Job drawing, mm, ordinate dimensions from the low corner. One solid piece. Coordinates: 2 decimals unless noted, no trailing zeros. Order: outer loops, then holes, each group sorted by start corner. A loop starts at its lowest first (then second) coordinate and runs counter-clockwise, first axis right, second up. Notation, with made-up numbers: (87.5, 36.5) - (93.5, 36.5) arc R23 ccw to (93.5, 69.5) - close; hole circle Ø7 at (-37.5, 64.5). An arc over 180 degrees is marked (long way). Write each question's results on one line, items separated by ' | '. Start each with the question number.
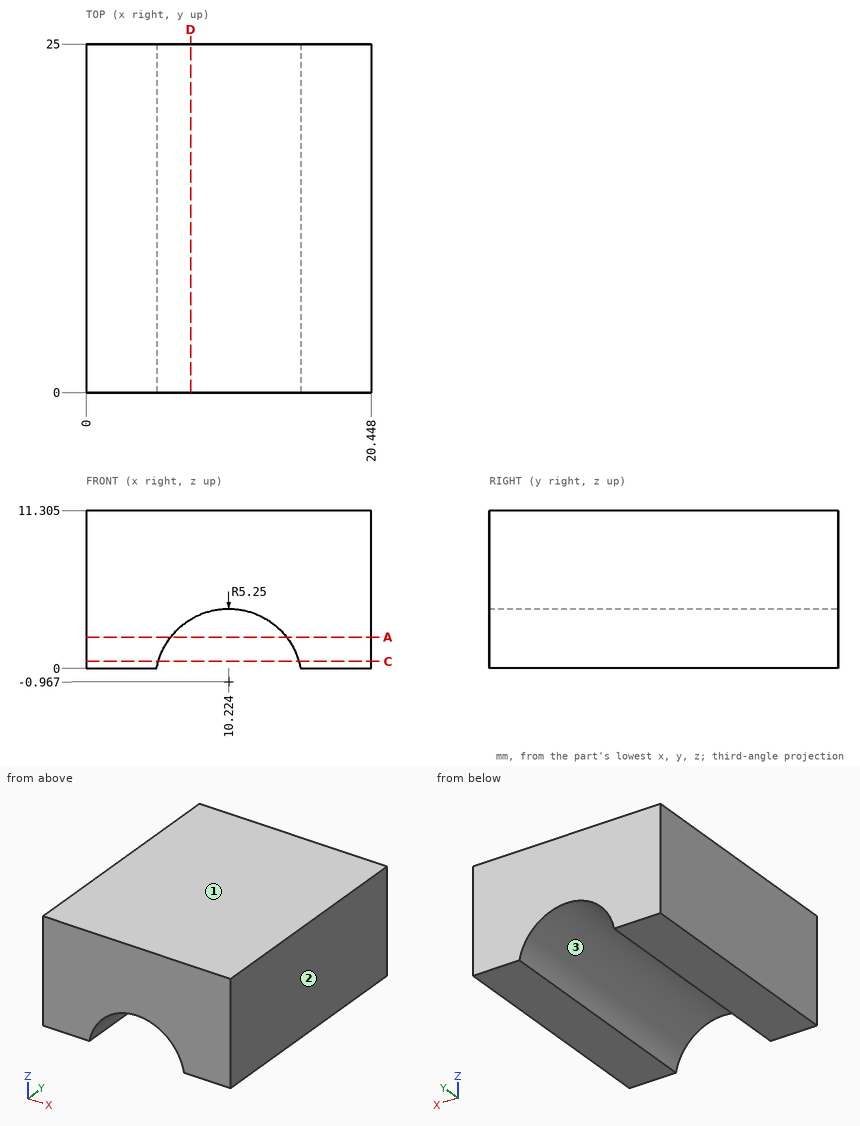
Item 1: Slice it at A-A (z = 2.25). Write the cut outline in (x, y) (1 decimal).
Item 2: Slice it at D-D (x = 7.5). Write the cut outline in (y, z) (1 decimal), then the cut area to 3 significant figures.
Item 3: Pull direction X, two halves, no side cores. Call the marked faces 1, 2 and 3: released by +X, released by -X, zero draft, split by the parting line, or undercut.
Item 4: Probe probe 1 along X at (y, z) = (4.25, 0.75) (1 decimal); probe 2 along Z at (x, y) = (10.25, 9) (1 decimal); probe 3 along X at (y, z) = (6.5, 1.5). List the from-to ranges inside material, lowest first.
Item 5: Slice it at C-C (z = 0.5). Write the cut outline in (x, y) (1 decimal).
Resolved:
1) outline: (0, 0) - (6.1, 0) - (6.1, 25) - (0, 25) - close; (14.4, 0) - (20.4, 0) - (20.4, 25) - (14.4, 25) - close
2) outline: (0, 3.5) - (25, 3.5) - (25, 11.3) - (0, 11.3) - close | area: 195 mm^2
3) face 1: zero draft | face 2: released by +X | face 3: undercut
4) probe 1: 0 to 5.3, 15.2 to 20.4 | probe 2: 4.3 to 11.3 | probe 3: 0 to 5.59, 14.86 to 20.45
5) outline: (0, 0) - (5.2, 0) - (5.2, 25) - (0, 25) - close; (15.3, 0) - (20.4, 0) - (20.4, 25) - (15.3, 25) - close
